Here's how the part is built. I have some questions about the finished solid (model axes, mm). Face numbers are marked on the shaded views. A direction names the side the tool comes from. Coordinates: 2 decimals unless noted, no trailing zeros. Write each loop counter-clockwise with the first axis right and the second up, starting at its lowest first coordinate (ties: lowest second). Pieces come first, ordered by that corner, then holes.
Item 1: For the marked faces 1 and 2, which set-ups out of +Z, -Z, +X, -X, +Y, -Y let a thin tool reach every point of the face, with its end or its side?
Item 2: I'm going to push flat-ended pins straight in: pin 1 Ø13 at (y, z) = (0, 0) entering from -X; pin 2 Ø5 at (x, z) = (8, -17.5) entering from +Y; pin 3 Ø8 at (x, y) = (2.5, -11) entering from -Z; pin 4 Ø6 at (x, z) = (4.5, 26.5) entering from +Y. Where does each tip first touch, or does it pass through?
Item 3: If I drill on line 1 (X direction, y = -12, z = 32.5); line 2 (Y direction, x = 6, z = 0); line 3 (Y direction, x = 9, z = 0), over which ranges is the centre line in solid material (lowest first)?
Item 4: We'd pull the mould along Y, two halves only. Please class the marked faces 3 and 4: +Y half, -Y half, draft (parallel to the pull), parting line (faces both ways), or undercut.
Item 5: If we section it at A-A (x = 10.5): Please give me the cut outline in (y, z).
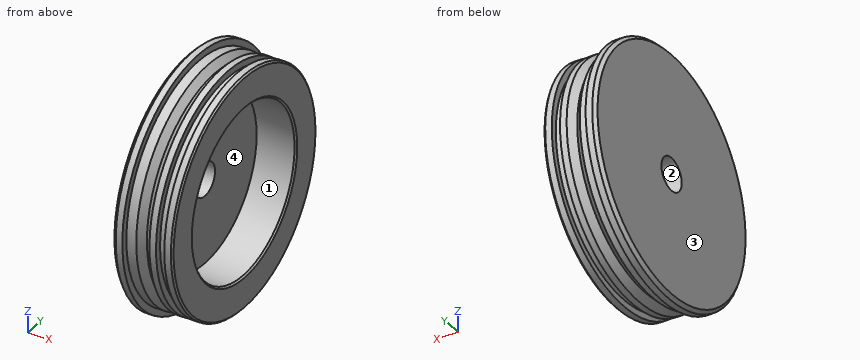
from build123d import *

# Parameters (mm, degrees)
SKETCH_2_R          = 5
CUT_EXTRUDE_1_DEPTH = 10


with BuildPart() as part:
    # Эскиз1 → Повернуть1 (revolve)
    with BuildSketch(Plane.XY, mode=Mode.PRIVATE) as revolve_1_sk:
        Polygon((-5, 0), (-5, 36.5), (-4, 37.5), (-2, 37.5), (-2, 35.5), (1, 35.5), (3, 33.5), (5, 35.5), (7, 35.5), (7, 33.5), (9.5, 33.5), (9.5, 35.5), (11.5, 35.5), (12, 35), (12, 26), (11.5, 25.5), (0, 25.5), (0, 0), align=None)
    revolve(revolve_1_sk.sketch.rotate(Axis((0, 0, 0), (1, 0, 0)), 90), axis=Axis((0, 0, 0), (1, 0, 0)))

    # Эскиз2 → Вырез-Вытянуть1 (cut)
    with BuildSketch(Plane.ZY.offset(5)):
        Circle(SKETCH_2_R)
    extrude(amount=-CUT_EXTRUDE_1_DEPTH, mode=Mode.SUBTRACT)


solid = part.part
Answer list:
1. face 1: +X
1. face 2: +X, -X
2. pin 1: stops at x = -5
2. pin 2: stops at y = 32.08
2. pin 3: stops at z = -34.74
2. pin 4: stops at y = 26.57
3. line 1: x = -5 to 1.86, 4.14 to 7, 9.5 to 12
3. line 2: y = -35.5 to -25.5, 25.5 to 35.5
3. line 3: y = -33.5 to -25.5, 25.5 to 33.5
4. face 3: draft
4. face 4: undercut
5. outline: circle Ø71 at (0, 0); hole circle Ø51 at (0, 0)
